```python
from build123d import *

# Parameters (mm, degrees)
SKETCH1_W             = 11
SKETCH1_H             = 31
BOSS_EXTRUDE1_DEPTH   = 3.81
SKETCH1_W_2           = 31
SKETCH1_H_2           = 11
BOSS_EXTRUDE1_2_DEPTH = 3.81
BOSS_EXTRUDE1_3_DEPTH = 3.81
BOSS_EXTRUDE1_4_DEPTH = 3.81
BOSS_EXTRUDE1_5_DEPTH = 3.81
SKETCH1_W_3           = 80
SKETCH1_H_3           = 100
SKETCH1_W_4           = 78.5
SKETCH1_H_4           = 98.5
BOSS_EXTRUDE1_6_DEPTH = 3.81
SKETCH3_W             = 80
SKETCH3_H             = 100
SKETCH3_W_2           = 31
SKETCH3_H_2           = 11
SKETCH3_W_3           = 11
SKETCH3_H_3           = 31
BOSS_EXTRUDE2_DEPTH   = 1.5875
FILLET1_R             = 0.05
SKETCH9_W             = 80
SKETCH9_H             = 100
BOSS_EXTRUDE6_DEPTH   = 6.096


with BuildPart() as part:
    # Sketch1 → Boss-Extrude1 (new body)
    with BuildSketch(Plane.XY):
        Polygon((-26.313903431, 0.439060111), (-31.5, 2.5), (-31.5, 35.5), (-25.083245041, 38.05), (-18.5, 35.5), (-18.5, 2.5), (-23.846750882, 0.428952262), (-23.616775358, 0.03062297), (-23.846750882, -0.367706323), (-18.5, -2.438754061), (-18.5, -35.438754061), (-25.083245041, -37.988754061), (-31.5, -35.438754061), (-31.5, -2.438754061), (-26.313903431, -0.377814172), (-26.549714725, 0.03062297), align=None)
        with Locations((-25, -18.938754061)):
            Rectangle(SKETCH1_W, SKETCH1_H, mode=Mode.SUBTRACT)
        with Locations((-25, 19)):
            Rectangle(SKETCH1_W, SKETCH1_H, mode=Mode.SUBTRACT)
    extrude(amount=BOSS_EXTRUDE1_DEPTH)



with BuildPart() as body_2:
    # Sketch1 → Boss-Extrude1 2 (new body)
    with BuildSketch(Plane.XY):
        Polygon((-19.05, 0.03062297), (-16.5, 6.5), (16.5, 6.5), (19.05, 0.03062297), (16.5, -6.438754061), (-16.5, -6.438754061), align=None)
        Rectangle(SKETCH1_W_2, SKETCH1_H_2, mode=Mode.SUBTRACT)
    extrude(amount=BOSS_EXTRUDE1_2_DEPTH)


with BuildPart() as body_3:
    # Sketch1 → Boss-Extrude1 3 (new body)
    with BuildSketch(Plane.XY):
        Polygon((26.313903431, 0.439060111), (26.549714725, 0.03062297), (26.313903431, -0.377814172), (31.5, -2.438754061), (31.5, -35.438754061), (25.083245041, -37.988754061), (18.5, -35.438754061), (18.5, -2.438754061), (23.846750882, -0.367706323), (23.616775358, 0.03062297), (23.846750882, 0.428952262), (18.5, 2.5), (18.5, 35.5), (25.083245041, 38.05), (31.5, 35.5), (31.5, 2.5), align=None)
        with Locations((25, 19)):
            Rectangle(SKETCH1_W, SKETCH1_H, mode=Mode.SUBTRACT)
        with Locations((25, -18.938754061)):
            Rectangle(SKETCH1_W, SKETCH1_H, mode=Mode.SUBTRACT)
    extrude(amount=BOSS_EXTRUDE1_3_DEPTH)


with BuildPart() as body_4:
    # Sketch1 → Boss-Extrude1 4 (new body)
    with BuildSketch(Plane.XY):
        Polygon((-16.5, 31.52602227), (-19.05, 38.013011135), (-16.5, 44.5), (16.5, 44.5), (19.05, 38.013011135), (16.5, 31.52602227), align=None)
        with Locations((0, 38)):
            Rectangle(SKETCH1_W_2, SKETCH1_H_2, mode=Mode.SUBTRACT)
    extrude(amount=BOSS_EXTRUDE1_4_DEPTH)


with BuildPart() as body_5:
    # Sketch1 → Boss-Extrude1 5 (new body)
    with BuildSketch(Plane.XY):
        Polygon((16.5, -31.464776331), (19.05, -37.951765196), (16.5, -44.438754061), (-16.5, -44.438754061), (-19.05, -37.951765196), (-16.5, -31.464776331), align=None)
        with Locations((0, -37.938754061)):
            Rectangle(SKETCH1_W_2, SKETCH1_H_2, mode=Mode.SUBTRACT)
    extrude(amount=BOSS_EXTRUDE1_5_DEPTH)


with BuildPart() as body_6:
    # Sketch1 → Boss-Extrude1 6 (new body)
    with BuildSketch(Plane.XY):
        Rectangle(SKETCH1_W_3, SKETCH1_H_3)
        Rectangle(SKETCH1_W_4, SKETCH1_H_4, mode=Mode.SUBTRACT)
    extrude(amount=BOSS_EXTRUDE1_6_DEPTH)


with BuildPart() as part_1:
    add(part.part)

    add(body_2.part)  # Boss-Extrude2 merges body 2

    add(body_3.part)  # Boss-Extrude2 merges body 3

    add(body_4.part)  # Boss-Extrude2 merges body 4

    add(body_5.part)  # Boss-Extrude2 merges body 5

    add(body_6.part)  # Boss-Extrude2 merges body 6
    # Sketch3 → Boss-Extrude2 (add)
    with BuildSketch(Plane.XY.offset(3.81)):
        Rectangle(SKETCH3_W, SKETCH3_H)
        with Locations((0, -37.938754061)):
            Rectangle(SKETCH3_W_2, SKETCH3_H_2, mode=Mode.SUBTRACT)
        Rectangle(SKETCH3_W_2, SKETCH3_H_2, mode=Mode.SUBTRACT)
        with Locations((-25, -18.938754061)):
            Rectangle(SKETCH3_W_3, SKETCH3_H_3, mode=Mode.SUBTRACT)
        with Locations((-25, 19)):
            Rectangle(SKETCH3_W_3, SKETCH3_H_3, mode=Mode.SUBTRACT)
        with Locations((0, 38)):
            Rectangle(SKETCH3_W_2, SKETCH3_H_2, mode=Mode.SUBTRACT)
        with Locations((25, 19)):
            Rectangle(SKETCH3_W_3, SKETCH3_H_3, mode=Mode.SUBTRACT)
        with Locations((25, -18.938754061)):
            Rectangle(SKETCH3_W_3, SKETCH3_H_3, mode=Mode.SUBTRACT)
    extrude(amount=BOSS_EXTRUDE2_DEPTH)

    # Fillet1
    fillet1_edges = [part_1.edges().sort_by_distance(p)[0] for p in [
        (39.25, 49.25, 1.905),
        (39.25, -49.25, 1.905),
        (-39.25, -49.25, 1.905),
        (-39.25, 49.25, 1.905),
    ]]
    fillet(fillet1_edges, radius=FILLET1_R)

    # Sketch9 → Boss-Extrude6 (add)
    with BuildSketch(Plane(origin=(0, 0, 0), x_dir=(-1, 0, 0), z_dir=(0, 0, -1))):
        Rectangle(SKETCH9_W, SKETCH9_H)
        with BuildLine():
            Line((39.2, 49.25), (-39.2, 49.25))
            ThreePointArc((-39.2, 49.25), (-39.235355339, 49.235355339), (-39.25, 49.2))
            Line((-39.25, 49.2), (-39.25, -49.2))
            ThreePointArc((-39.25, -49.2), (-39.235355339, -49.235355339), (-39.2, -49.25))
            Line((-39.2, -49.25), (39.2, -49.25))
            ThreePointArc((39.2, -49.25), (39.235355339, -49.235355339), (39.25, -49.2))
            Line((39.25, -49.2), (39.25, 49.2))
            ThreePointArc((39.25, 49.2), (39.235355339, 49.235355339), (39.2, 49.25))
        make_face(mode=Mode.SUBTRACT)
    extrude(amount=BOSS_EXTRUDE6_DEPTH)


solid = part_1.part
```
The model under review builds one solid part; all positions refer to its coordinate system, in mm. A direction names the side the tool comes from. Round coordinates to 2 decimals unless told otherwise and drop trailing zeros. Write each loop counter-clockwise with the first axis right and the second up, starting at its lowest first coordinate (ties: lowest second). Pieces come first, ordered by that corner, then holes. Notation, with made-up numbers: (10.5, 0) - (43.5, 0) arc R38 cw to (43.5, 38) - close; hole circle Ø3 at (80.25, 6). An arc over 180 degrees is marked (long way). One line per question, with ' | ' between items.
Item 1: The part is to be moulded in two halves that separate along Y. For faces 3 (the face through (21.21, 1.45, 1.88)), 4 (the face through (-1, 12, 5.398)), say which applies: pulls with the +Y half, pulls with the -Y half, needs draft (parallel to the pull), parting line crosses it, or undercut.
Resolved:
face 3: undercut | face 4: needs draft
Item 2: For P1, Ø10.5, axis at x = -3.5, y = 2.5, coming from the -Z side, flat-tipped, find the tip position at first contact; note if it passes through.
Resolved:
P1: stops at z = 0
Item 3: For faces 1 (the face through (17.76, 41.3, 1.88)), 2 (the face through (25, 34.5, 3)), list the 3-axis set-ups (+Z, -Z, +X, -X, +Y, -Y) from which the entire face can be reached by the end or side of a thin tool; tool diameter is ignored.
Resolved:
face 1: -Z | face 2: +Z, -Z
Item 4: Add section B-B, the plane y = -36.5. Give the boundary of the cut face in (x, z), then the cut area to 3 significant figures.
Resolved:
outline: (-40, -6.1) - (-39.25, -6.1) - (-39.25, 3.81) - (-28.83, 3.81) - (-28.83, 0) - (-21.24, 0) - (-21.24, 3.81) - (-18.48, 3.81) - (-18.48, 0) - (-15.5, 0) - (-15.5, 5.4) - (-40, 5.4) - close; (15.5, 0) - (18.48, 0) - (18.48, 3.81) - (21.24, 3.81) - (21.24, 0) - (28.83, 0) - (28.83, 3.81) - (39.25, 3.81) - (39.25, -6.1) - (40, -6.1) - (40, 5.4) - (15.5, 5.4) - close | area: 173 mm2
Item 5: Add section A-A, the plane x = 0. State how many separate pieces and enclosed holes the cut face has, then the cut area to 3 significant figures.
Resolved:
separate pieces: 4 | enclosed holes: 0 | area: 144 mm2
Item 6: Add section D-D, the plane x = 34. Give the boundary of the cut face in (y, z).
Resolved:
outline: (-50, -6.1) - (-49.25, -6.1) - (-49.25, 3.81) - (49.25, 3.81) - (49.25, -6.1) - (50, -6.1) - (50, 5.4) - (-50, 5.4) - close
Item 7: To check wall thickness, follow probe 1 along X at (y, z) = (-22.5, 3); probe 2 along Y at (x, z) = (-24, 4.5); probe 3 along Y at (x, z) = (2, -3). State the ranges of each line that lie inside material, in increasing order.
Resolved:
probe 1: x = -40 to -39.25, -31.5 to -30.5, -19.5 to -18.5, 18.5 to 19.5, 30.5 to 31.5, 39.25 to 40 | probe 2: y = -50 to -34.44, -3.44 to 3.5, 34.5 to 50 | probe 3: y = -50 to -49.25, 49.25 to 50
Item 8: Add section C-C, the plane y = 24.5. Give the boundary of the cut face in (x, z), then the cut area to 3 significant figures.
Resolved:
outline: (-40, -6.1) - (-39.25, -6.1) - (-39.25, 3.81) - (-31.5, 3.81) - (-31.5, 0) - (-30.5, 0) - (-30.5, 5.4) - (-40, 5.4) - close; (-19.5, 0) - (-18.5, 0) - (-18.5, 3.81) - (18.5, 3.81) - (18.5, 0) - (19.5, 0) - (19.5, 5.4) - (-19.5, 5.4) - close; (30.5, 0) - (31.5, 0) - (31.5, 3.81) - (39.25, 3.81) - (39.25, -6.1) - (40, -6.1) - (40, 5.4) - (30.5, 5.4) - close | area: 122 mm2
